from build123d import *

# Parameters (mm, degrees)
PAD_DEPTH       = 3.7
SKETCH001_W     = 2.7
SKETCH001_H     = 1.7
POCKET_DEPTH    = 2
SKETCH002_R     = 1.3
PAD001_DEPTH    = 1
SKETCH003_W     = 1.5
SKETCH003_H     = 3.7
PAD002_DEPTH    = 0.4
POCKET001_DEPTH = 5
SKETCH005_R     = 1.3
PAD003_DEPTH    = 1
SKETCH006_W     = 1.5
SKETCH006_H     = 3.7
PAD004_DEPTH    = 0.4
POCKET002_DEPTH = 5
SKETCH008_W     = 4.7
SKETCH008_H     = 3.7
POCKET003_DEPTH = 0.4
SKETCH009_W     = 1.3
SKETCH009_H     = 3.7
POCKET004_DEPTH = 0.7
SKETCH010_W     = 2.5
SKETCH010_H     = 3.592296
POCKET005_DEPTH = 0.2
SKETCH011_W     = 2
SKETCH011_H     = 3.592296
POCKET006_DEPTH = 0.2


with BuildPart() as part:
    # Sketch → Pad (new body)
    with BuildSketch(Plane.XY):
        Polygon((0, 28), (0, 0), (4.7, 0), (4.7, 3.5), (1.3, 3.5), (1.3, 5.3), (5.8, 5.3), (5.8, 6.3), (1.3, 6.3), (1.3, 20.5), (5.8, 20.5), (5.8, 21.5), (1.3, 21.5), (1.3, 23.3), (5.8, 23.3), (5.8, 24.3), (1.3, 24.3), (1.3, 28), align=None)
    extrude(amount=PAD_DEPTH)

    # Sketch001 → Pocket (cut)
    with BuildSketch(Plane.XZ):
        with Locations((2.35, 1.85)):
            Rectangle(SKETCH001_W, SKETCH001_H)
    extrude(amount=-POCKET_DEPTH, mode=Mode.SUBTRACT)

    # Sketch002 → Pad001 (new body)
    with BuildSketch(Plane.XZ.offset(-5.3)):
        with Locations((4.4, 1.85)):
            Circle(SKETCH002_R)
    extrude(amount=PAD001_DEPTH)

    # Sketch003 → Pad002 (new body)
    with BuildSketch(Plane.XZ.offset(-5.3)):
        with Locations((5.05, 1.85)):
            Rectangle(SKETCH003_W, SKETCH003_H)
    extrude(amount=PAD002_DEPTH)

    # Sketch004 → Pocket001 (cut)
    with BuildSketch(Plane.XY.offset(3.7)):
        Polygon((5.8, 5.3), (4.3, 4.3), (5.8, 4.3), align=None)
    extrude(amount=-POCKET001_DEPTH, mode=Mode.SUBTRACT)

    # Sketch005 → Pad003 (new body)
    with BuildSketch(Plane.XZ.offset(-23.3)):
        with Locations((4.4, 1.85)):
            Circle(SKETCH005_R)
    extrude(amount=PAD003_DEPTH)

    # Sketch006 → Pad004 (new body)
    with BuildSketch(Plane.XZ.offset(-23.3)):
        with Locations((5.05, 1.85)):
            Rectangle(SKETCH006_W, SKETCH006_H)
    extrude(amount=PAD004_DEPTH)

    # Sketch007 → Pocket002 (cut)
    with BuildSketch(Plane.XY.offset(3.7)):
        Polygon((5.8, 23.3), (4.3, 22.3), (5.8, 22.3), align=None)
    extrude(amount=-POCKET002_DEPTH, mode=Mode.SUBTRACT)

    # Sketch008 → Pocket003 (cut)
    with BuildSketch(Plane.XZ):
        with Locations((2.35, 1.85)):
            Rectangle(SKETCH008_W, SKETCH008_H)
    extrude(amount=-POCKET003_DEPTH, mode=Mode.SUBTRACT)

    # Sketch009 → Pocket004 (cut)
    with BuildSketch(Plane(origin=(0, 28, 0), x_dir=(-1, 0, 0), z_dir=(0, 1, 0))):
        with Locations((-0.65, 1.85)):
            Rectangle(SKETCH009_W, SKETCH009_H)
    extrude(amount=-POCKET004_DEPTH, mode=Mode.SUBTRACT)

    # Sketch010 → Pocket005 (cut)
    with BuildSketch(Plane.XZ.offset(-4.3)):
        with Locations((4.05, 1.85)):
            Rectangle(SKETCH010_W, SKETCH010_H)
    extrude(amount=-POCKET005_DEPTH, mode=Mode.SUBTRACT)

    # Sketch011 → Pocket006 (cut)
    with BuildSketch(Plane.XZ.offset(-22.3)):
        with Locations((3.8, 1.85)):
            Rectangle(SKETCH011_W, SKETCH011_H)
    extrude(amount=-POCKET006_DEPTH, mode=Mode.SUBTRACT)


solid = part.part
Design review of the part built by this model. Coordinates are the model's own, in mm. A direction names the side the tool comes from. Coordinates: 2 decimals unless noted, no trailing zeros. Order: outer loops, then holes, each group sorted by start corner. A loop starts at its lowest first (then second) coordinate and runs counter-clockwise, first axis right, second up. Notation, with made-up numbers: (73.25, -14.75) -> (91.25, -14.75) arc R29 cw to (91.25, 12.25) -> close; hole circle Ø10 at (-17, 80.5). An arc over 180 degrees is marked (long way). Use one line per item in the form item = value. Start each with the question number.
(1) For probe 1 along Y at (x, z) = (3.5, 3.65); probe 2 along Y at (x, z) = (4.2, 0.7); probe 3 along X at (y, z) = (23, 3.25), list the stretches that pass through material, from the lowest coordinate up.
(2) The part is to be moulded in two halves that separate along X. For faces 6 (the flat face through (4, 21.5, 2)), 7 (the flat face through (4.7, 2, 2)), 8 (the flat face through (1, 1, 2)), say which applies: +X half, -X half, draft (parallel to the pull), parting line (faces both ways), or undercut.
(3) For faces 1 (the flat face through (1.3, 4, 2)), 2 (the flat face through (4, 20.5, 2)), 3 (the flat face through (4, 24.3, 2)), 4 (the flat face through (2, 1, 2.7)), 5 (the cylindrical face through (3.1, 4.9, 1.9)), list the 3-axis set-ups (+Z, -Z, +X, -X, +Y, -Y) from which the entire face can be reached by the end or side of a thin tool; tool diameter is ignored.
(4) Add section B-B on y = 2.75. State the section outline as (x, z) points.
(5) Add section A-A on z = 1.85. State the section outline as (x, y) points.
(6) Insertion check: pin 1 (0.9 mm diameter, centred on x = 3, z = 2, fed in from -Y); pin 2 (1.1 mm diameter, centred on x = 4, z = 2.5, fed in from +Y); pin 3 (1 mm diameter, centred on y = 16.5, z = 3, fed in from +X). Each pin has a flat end and moves straight along its axis. Give the tip position at first contact, or say it passes through.
Answer block:
q1.probe_1 = 0.4 to 3.5, 5.3 to 6.3, 20.5 to 21.5, 23.3 to 24.3
q1.probe_2 = 0.4 to 3.5, 4.5 to 6.3, 20.5 to 21.5, 22.5 to 24.3
q1.probe_3 = 0 to 1.3, 4.3 to 5.35
q2.face_6 = draft
q2.face_7 = +X half
q2.face_8 = undercut
q3.face_1 = +Z, -Z
q3.face_2 = +Z, -Z, +X
q3.face_3 = +Z, -Z, +X, +Y
q3.face_4 = -Y
q3.face_5 = none
q4.outline = (0, 0) -> (4.7, 0) -> (4.7, 3.7) -> (0, 3.7) -> close
q5.outline = (0, 0.4) -> (1, 0.4) -> (1, 2) -> (3.7, 2) -> (3.7, 0.4) -> (4.7, 0.4) -> (4.7, 3.5) -> (1.3, 3.5) -> (1.3, 5.3) -> (3.1, 5.3) -> (3.1, 4.5) -> (4.6, 4.5) -> (5.8, 5.3) -> (5.8, 6.3) -> (1.3, 6.3) -> (1.3, 20.5) -> (5.8, 20.5) -> (5.8, 21.5) -> (1.3, 21.5) -> (1.3, 23.3) -> (3.1, 23.3) -> (3.1, 22.5) -> (4.6, 22.5) -> (5.8, 23.3) -> (5.8, 24.3) -> (1.3, 24.3) -> (1.3, 27.3) -> (0, 27.3) -> close
q6.pin_1 = 2
q6.pin_2 = 24.3
q6.pin_3 = 1.3
